Design review of the part built by this model. Coordinates are the model's own, in mm. A direction names the side the tool comes from. Give positions to 0.01 mm unless a question says otherwise; leave off trailing zeros. Loops run counter-clockwise (first coordinate to the right, second up) from the corner with the lowest first, then second, coordinate; pieces in that order, holes last. Notation, with made-up numbers: (36, 19.5) -> (82, 19.5) arc R24 ccw to (82, 43.5) -> close; hole circle Ø6 at (-22, 55.5). An arc over 180 degrees is marked (long way). Use a Markdown table: item, result. Add a question column.
1. To check wall thickness, follow line 1 (Y direction, x = 21, z = 111); line 2 (X direction, y = -42.5, z = 24.5); line 3 (X direction, y = -20.5, z = 25). State the ranges of each line that lie inside material, in increasing order.
2. Add section A-A (x = 24). Count the separate pieces of the cut face and the enclosed holes in it, and give its area (3 significant figures).
3. Add section C-C (y = -28). State the section outline as (x, z) points.
4. Add section D-D (y = -57). State the section outline as (x, z) points.
5. For pin 1 Ø14.5 at (x, z) = (25.5, 111.5) entering from -Y; pin 2 Ø2 at (x, z) = (9, 103.5) entering from -Y; pin 3 Ø9 at (x, z) = (24, 182) entering from -Y; pin 4 Ø2 at (y, z) = (-26.5, 151) entering from +X, all flat-tipped, find the tip position at first contact; note any pin that passes through.
6. Add section B-B (z = 52). State the section outline as (x, y) points.
7. Draft analysis for pull direction Y (two halves, no side actions). For faces 4 (the flat face through (16, 0, 118)), 5 (the cylindrical face through (10.96, -17.9, 118.32)), 6 (the cylindrical face through (25.08, -1.97, 82.12)), state which applies: pulls with the +Y half, pulls with the -Y half, needs draft (parallel to the pull), parting line crosses it, or undercut.
8. For faces 1 (the flat face through (20, -4, 118)), 2 (the flat face through (33, -2, 118)), 3 (the flat face through (6, -35, 118)), list the 3-axis set-ups (+Z, -Z, +X, -X, +Y, -Y) from which the entire face can be reached by the end or side of a thin tool; tool diameter is ignored.
Autodesk Fusion 360 part; units mm, degrees
sketch "Sketch1" plane through (0, 0, 0) normal (0, 0, 1) x (1, 0, 0) in component "Component"
  line L0 (0, 0) -> (6, 0)
  line L1 (6, 0) -> (6, -67)
  line L2 (6, -67) -> (0, -67)
  line L3 (0, -67) -> (0, 0)
  line L4 (6, 0) -> (18, 0)
  line L5 (18, 0) -> (18, -4)
  line L6 (18, -4) -> (6, -4)
  line L7 (6, -4) -> (6, 0)
  line L8 (8.0693, -4) -> (8.0693, -32) construction
  arc A0 (12, -4) -> (8.0693, -32) centre (59.8982, -25) ccw
  arc A1 (15.1021, -4) -> (10.8522, -32) centre (61.2859, -25.3325) ccw
  line L9 (8.0693, -32) -> (10.8522, -32)
  dimension "d1" = 6
  dimension "d2" = 67
  dimension "d3" = 12
  dimension "d4" = 4
  dimension "d5" = 28
extrude "Extrude1" add sketch "Sketch1" along normal blind 240 in component "Component"
sketch "Sketch2" plane through (0, 0, 0) normal (0, 1, 0) x (-1, 0, 0) in component "Component"
  line L0 (-18, 0) -> (0, 0)
  line L1 (0, 0) -> (0, 240)
  line L2 (0, 240) -> (-18, 240)
  line L3 (-18, 240) -> (-18, 0)
  circle A0 centre (-24, 17) radius 5
  line L4 (-9, 47) -> (-24, 52) construction
  circle A1 centre (-24, 52) radius 5
  circle A2 centre (-24, 87) radius 5
  circle A3 centre (-24, 122) radius 5
  circle A4 centre (-24, 152) radius 5
  circle A5 centre (-24, 182) radius 5
  circle A6 centre (-24, 212) radius 5
  dimension "d10" = 10
  dimension "d12" = 10
  dimension "d14" = 10
  dimension "d16" = 10
  dimension "d18" = 10
  dimension "d20" = 10
  dimension "d22" = 10
sketch "Sketch3" plane through (0, 0, 0) normal (0, 0, 1) x (1, 0, 0) in component "Component"
  line L0 (18, 0) -> (33, 0)
  line L1 (18, -4) -> (33, -4)
  line L2 (33, -4) -> (33, 0)
  line L3 (18, 0) -> (18, -4)
  dimension "d23" = 15
extrude "Extrude2" add sketch "Sketch3" along normal blind 240 in component "Component"
extrude "Extrude3" cut sketch "Sketch2" against normal blind 20 contours A0 | A1 | A2 | A3 | A4 | A5 | A6 in component "Component"
component "Component" placed x (1, 0, 0) y (0, 1, 0) z (0, 0, 1) at (0, 0, 0)
Taken from the geometry:
| question | item | result |
|---|---|---|
| 1 | line 1 | y = -4 to 0 |
| 1 | line 2 | x = 0 to 6 |
| 1 | line 3 | x = 0 to 6, 7.79 to 10.64 |
| 2 | separate pieces | 8 |
| 2 | enclosed holes | 0 |
| 2 | area | 680 mm^2 |
| 3 | outline | (0, 0) -> (6, 0) -> (6, 240) -> (0, 240) -> close; (7.68, 0) -> (10.48, 0) -> (10.48, 240) -> (7.68, 240) -> close |
| 4 | outline | (0, 0) -> (6, 0) -> (6, 240) -> (0, 240) -> close |
| 5 | pin 1 | stops at y = -4 |
| 5 | pin 2 | stops at y = -32 |
| 5 | pin 3 | passes through |
| 5 | pin 4 | stops at x = 10.46 |
| 6 | outline | (0, -67) -> (6, -67) -> (6, -4) -> (12, -4) arc R52.3 ccw to (8.07, -32) -> (10.85, -32) arc R50.87 cw to (15.1, -4) -> (19, -4) -> (19, 0) -> (0, 0) -> close; (29, -4) -> (33, -4) -> (33, 0) -> (29, 0) -> close |
| 7 | face 4 | pulls with the +Y half |
| 7 | face 5 | undercut |
| 7 | face 6 | needs draft |
| 8 | face 1 | +Z, -Z, +X, -Y |
| 8 | face 2 | +Z, -Z, +X, +Y, -Y |
| 8 | face 3 | +Z, -Z, -Y |
